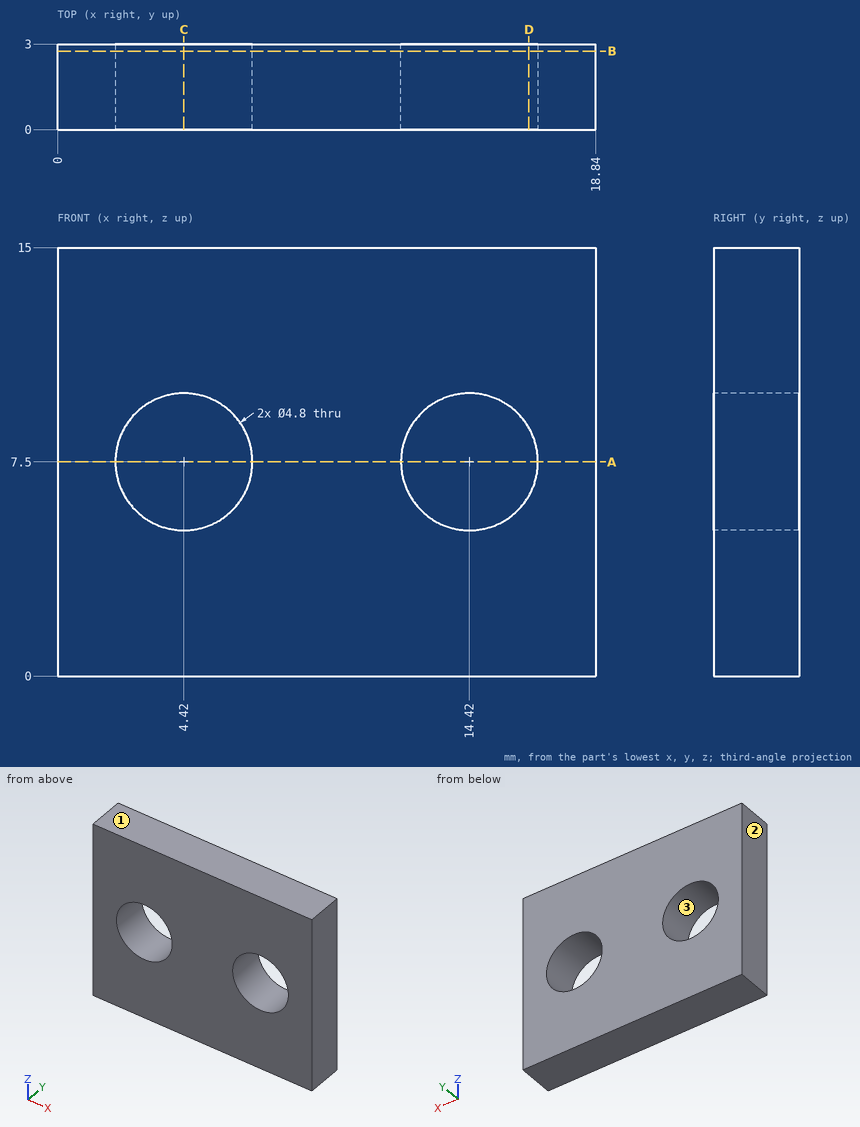
The drawing under review shows one solid part. Ordinate dimensions are in mm from its lowest x, y, z. Give positions to 0.01 mm unless a question says otherwise; leave off trailing zeros. Loops run counter-clockwise (first coordinate to the right, second up) from the corner with the lowest first, then second, coordinate; pieces in that order, holes last. Notation, with made-up numbers: M 69.5,51 L 122.5,51 A22 cw 122.5,88 Z; hole C 41.5,27.5 d9. An arc over 180 degrees is marked long. One line per item, written item: value. Start each with the question number.
Q1. Add section B-B (y = 2.75). Give the boundary of the cut face in (x, z), and give its area (3 significant figures).
Q2. For L1, parallel to Z at x = 14.42, y = 2.15; L2, parallel to X at y = 2.6, z = 6.5; L3, parallel to Z at x = 15, y = 1.35, list the stretches that pass through material, from the lowest coordinate up.
Q3. Draft analysis for pull direction Z (two halves, no side actions). For the marked faces 1, 2 and 3, state which applies: released by +Z, released by -Z, zero draft, split by the parting line, or undercut.
Q4. Add section A-A (z = 7.5). Give the boundary of the cut face in (x, y), and give its area (3 significant figures).
Q5. Add section D-D (x = 16.5). Give the boundary of the cut face in (y, z).
Q6. Add section C-C (x = 4.42). Give the boundary of the cut face in (y, z), and give its area (3 significant figures).
Reply:
1. outline: M 0,0 L 18.84,0 L 18.84,15 L 0,15 Z; hole C 4.42,7.5 d4.8; hole C 14.42,7.5 d4.8
1. area: 246 mm²
2. L1: 0 to 5.1, 9.9 to 15
2. L2: 0 to 2.24, 6.6 to 12.24, 16.6 to 18.84
2. L3: 0 to 5.17, 9.83 to 15
3. face 1: released by +Z
3. face 2: zero draft
3. face 3: undercut
4. outline: M 0,0 L 2.02,0 L 2.02,3 L 0,3 Z; M 6.82,0 L 12.02,0 L 12.02,3 L 6.82,3 Z; M 16.82,0 L 18.84,0 L 18.84,3 L 16.82,3 Z
4. area: 27.7 mm²
5. outline: M 0,0 L 3,0 L 3,6.3 L 0,6.3 Z; M 0,8.7 L 3,8.7 L 3,15 L 0,15 Z
6. outline: M 0,0 L 3,0 L 3,5.1 L 0,5.1 Z; M 0,9.9 L 3,9.9 L 3,15 L 0,15 Z
6. area: 30.6 mm²
